Design review of the part built by this model. Coordinates are the model's own, in mm. A direction names the side the tool comes from. Coordinates: 2 decimals unless noted, no trailing zeros. Loops run counter-clockwise (first coordinate to the right, second up) from the corner with the lowest first, then second, coordinate; pieces in that order, holes last. Notation, with made-up numbers: (-17.5, -30.5) - (1.5, -30.5) arc R21 cw to (1.5, -12.5) - close; hole circle Ø11 at (3.5, 1.25). An arc over 180 degrees is marked (long way). Answer in a Markdown table with one row per item. Add a question column.
(1) We need section A-A, the plane x = 44.5. Write out the cut boundary in (y, z), plus the area to 3 significant figures.
(2) For faces 1 (the face through (1, -6, -1)), 2 (the face through (81.085, 2.958, 77.54)), 3 (the face through (0, -12, -21)), 4 (the face through (-28.25, -11.92, -0.33)), 5 (the face through (99.04, 2.96, -55.97)), list the 3-axis set-ups (+Z, -Z, +X, -X, +Y, -Y) from which the entire face can be reached by the end or side of a thin tool; tool diameter is ignored.
(3) We need section D-D, the plane z = -113. Write out the cut boundary in (x, y), plus the area to 3 significant figures.
(4) We need section B-B, the plane z = -78. Write out the cut boundary in (x, y).
(5) Clearance check with flat-ended pins moving along their axes: pin 1 (1.8 mm diameter, centred on y = -1.5, z = 1, fed in from +X); pin 2 (6 mm diameter, centred on x = 51, z = 20.5, fed in from -Y); pin 3 (1.8 mm diameter, centred on x = -21, y = -6.5, fed in from -Z). State where each tip first meets the part, or that it passes through.
(6) The part is to be moulded in two halves that separate along Z. For faces 6 (the face through (28.25, -11.92, 0.33)), 7 (the face through (-100.751, 2.958, -57.284)), 8 (the face through (100, 0, 78)), say which applies: released by +Z, released by -Z, zero draft, split by the parting line, or undercut.
(7) We need section C-C, the plane x = 0. Write out the cut boundary in (y, z).
(8) To check wall thickness, follow L1, parallel to X at y = -4.75, z = 1; L2, parallel to Z at x = 8, y = -16.35; L3, parallel to Y at x = -136, z = 96. State the ranges of each line that lie inside material, in increasing order. Write a range as [from, to].
from build123d import *

# Parameters (mm, degrees)
SALIENTE_EXTRUIR1_DEPTH = 6
SALIENTE_EXTRUIR2_DEPTH = 12
CROQUIS7_R              = 40
SALIENTE_EXTRUIR5_DEPTH = 6
SALIENTE_EXTRUIR3_DEPTH = 6
CROQUIS6_R              = 1.75
SALIENTE_EXTRUIR4_DEPTH = 6
CROQUIS8_W              = 6
CROQUIS8_H              = 6
CORTAR_EXTRUIR1_DEPTH   = 31


with BuildPart() as part:
    # Croquis1 → Saliente-Extruir1 (new body)
    with BuildSketch(Plane(origin=(0, 0, 0), x_dir=(1, 0, 0), z_dir=(0, 1, 0))):
        with BuildLine():
            Line((-161, 103.5), (-38.791887254, 9.756509788))
            ThreePointArc((-38.791887254, 9.756509788), (-40, 0), (-38.791887254, -9.756509788))
            Line((-38.791887254, -9.756509788), (-161, -103.5))
            Line((-161, -103.5), (-161, -123.5))
            Line((-161, -123.5), (-141, -123.5))
            Line((-141, -123.5), (-22.823766962, -32.84928708))
            ThreePointArc((-22.823766962, -32.84928708), (0, -40), (22.823766962, -32.84928708))
            Line((22.823766962, -32.84928708), (141, -123.5))
            Line((141, -123.5), (161, -123.5))
            Line((161, -123.5), (161, -103.5))
            Line((161, -103.5), (38.791887254, -9.756509788))
            ThreePointArc((38.791887254, -9.756509788), (40, 0), (38.791887254, 9.756509788))
            Line((38.791887254, 9.756509788), (161, 103.5))
            Line((161, 103.5), (161, 123.5))
            Line((161, 123.5), (141, 123.5))
            Line((141, 123.5), (22.823766962, 32.84928708))
            ThreePointArc((22.823766962, 32.84928708), (0, 40), (-22.823766962, 32.84928708))
            Line((-22.823766962, 32.84928708), (-141, 123.5))
            Line((-141, 123.5), (-161, 123.5))
            Line((-161, 123.5), (-161, 103.5))
        make_face()
    extrude(amount=SALIENTE_EXTRUIR1_DEPTH)

    # Croquis4 → Saliente-Extruir2 (add)
    with BuildSketch(Plane(origin=(0, 0, 0), x_dir=(1, 0, 0), z_dir=(0, 1, 0))):
        Polygon((-161, 103.5), (-161, 123.5), (-141, 123.5), (-141, 129.5), (-167, 129.5), (-167, 103.5), align=None)
        Polygon((-161, -103.5), (-161, -123.5), (-141, -123.5), (-141, -129.5), (-167, -129.5), (-167, -103.5), align=None)
        Polygon((167, -103.5), (161, -103.5), (161, -123.5), (141, -123.5), (141, -129.5), (167, -129.5), align=None)
        Polygon((167, 103.5), (161, 103.5), (161, 123.5), (141, 123.5), (141, 129.5), (167, 129.5), align=None)
    extrude(amount=SALIENTE_EXTRUIR2_DEPTH)

    # Croquis7 → Saliente-Extruir5 (add)
    with BuildSketch(Plane(origin=(0, 0, 0), x_dir=(-1, 0, 0), z_dir=(0, -1, 0))):
        Circle(CROQUIS7_R)
    extrude(amount=SALIENTE_EXTRUIR5_DEPTH)

    # Croquis5 → Saliente-Extruir3 (add)
    with BuildSketch(Plane.XZ.offset(6)):
        with BuildLine():
            Line((18.896097481, -21), (-18.896097481, -21))
            ThreePointArc((-18.896097481, -21), (-28.25, 0), (-18.896097481, 21))
            Line((-18.896097481, 21), (-13.25, 21))
            Line((-13.25, 21), (-13.25, -11))
            Line((-13.25, -11), (13.25, -11))
            Line((13.25, -11), (13.25, 21))
            Line((13.25, 21), (18.896097481, 21))
            ThreePointArc((18.896097481, 21), (28.25, 0), (18.896097481, -21))
        make_face()
    extrude(amount=SALIENTE_EXTRUIR3_DEPTH)

    # Croquis6 → Saliente-Extruir4 (add)
    with BuildSketch(Plane.XZ.offset(12)):
        with BuildLine():
            Line((-18.896097481, 21), (-13.25, 21))
            Line((-13.25, 21), (-13.25, 3.5))
            ThreePointArc((-13.25, 3.5), (-13.103553391, 3.146446609), (-12.75, 3))
            Line((-12.75, 3), (12.75, 3))
            ThreePointArc((12.75, 3), (13.103553391, 3.146446609), (13.25, 3.5))
            Line((13.25, 3.5), (13.25, 21))
            Line((13.25, 21), (18.896097481, 21))
            ThreePointArc((18.896097481, 21), (28.25, 0), (18.896097481, -21))
            Line((18.896097481, -21), (-18.896097481, -21))
            ThreePointArc((-18.896097481, -21), (-28.25, 0), (-18.896097481, 21))
        make_face()
        with Locations((-8, -5.75)):
            Circle(CROQUIS6_R, mode=Mode.SUBTRACT)
        with Locations((8, -5.75)):
            Circle(CROQUIS6_R, mode=Mode.SUBTRACT)
    extrude(amount=SALIENTE_EXTRUIR4_DEPTH)

    # Croquis8 → Cortar-Extruir1 (cut, through all)
    with BuildSketch(Plane.XZ.offset(18)):
        with Locations((-20, 0)):
            Rectangle(CROQUIS8_W, CROQUIS8_H)
        with Locations((20, 0)):
            Rectangle(CROQUIS8_W, CROQUIS8_H)
    extrude(amount=-CORTAR_EXTRUIR1_DEPTH, mode=Mode.SUBTRACT)


solid = part.part
Responses:
| question | item | result |
|---|---|---|
| 1 | outline | (0, -49.48) - (6, -49.48) - (6, -14.14) - (0, -14.14) - close; (0, 14.14) - (6, 14.14) - (6, 49.48) - (0, 49.48) - close |
| 1 | area | 424 mm2 |
| 2 | face 1 | none |
| 2 | face 2 | +Z, +Y, -Y |
| 2 | face 3 | -Z, +X, -X, -Y |
| 2 | face 4 | -X, -Y |
| 2 | face 5 | +X, +Y, -Y |
| 3 | outline | (-167, 0) - (-127.31, 0) - (-127.31, 6) - (-161, 6) - (-161, 12) - (-167, 12) - close; (127.31, 0) - (167, 0) - (167, 12) - (161, 12) - (161, 6) - (127.31, 6) - close |
| 3 | area | 548 mm2 |
| 4 | outline | (-127.76, 0) - (-81.68, 0) - (-81.68, 6) - (-127.76, 6) - close; (81.68, 0) - (127.76, 0) - (127.76, 6) - (81.68, 6) - close |
| 5 | pin 1 | stops at x = 40 |
| 5 | pin 2 | stops at y = 0 |
| 5 | pin 3 | stops at z = -34.49 |
| 6 | face 6 | split by the parting line |
| 6 | face 7 | undercut |
| 6 | face 8 | zero draft |
| 7 | outline | (-18, -21) - (-6, -21) - (-6, -40) - (6, -40) - (6, 40) - (-6, 40) - (-6, -11) - (-12, -11) - (-12, 3) - (-18, 3) - close |
| 8 | L1 | x = [-39.99, -23], [-17, 17], [23, 39.99] |
| 8 | L2 | z = [-21, -7.5], [-4, 3] |
| 8 | L3 | y = [0, 6] |
